Verification items for the finished model (mm, model axes). Face numbers are marked on the shaded views. A direction names the side the tool comes from. Give positions to 0.01 mm unless a question says otherwise; leave off trailing zeros. Loops run counter-clockwise (first coordinate to the right, second up) from the corner with the lowest first, then second, coordinate; pieces in that order, holes last. Notation, with made-up numbers: (15.25, 34) - (48.25, 34) arc R27 ccw to (48.25, 51) - close; hole circle Ø3 at (-16, -17). An arc over 180 degrees is marked (long way). One line per item, written item: value. Start each with the question number.
1. Mould release check, pull along Y, two halves, no side actions. Record for the marked faces 4, 5 and 6: pulls with the +Y half, pulls with the -Y half, needs draft (parallel to the pull), parting line crosses it, or undercut.
2. Sectioned sample at C-C (y = 28.5). Record the cut outline in (x, z), plus the area to 3 significant figures.
3. Sectioned sample at D-D (y = 18). Record the cut outline in (x, z).
4. Scan lines: L1, parallel to Z at x = 60, y = 20.5; L2, parallel to X at y = 4, z = 28; L3, parallel to Z at x = 39, y = 7.5. Record each from-to range of solid material in increasing order. Write a range as [from, to].
5. Access from +Z, -Z, +X, -X, +Y, -Y to the whole of each face (thin tool, end or side, straight path). Record for the marked faces 1, 2 and 3.
6. Gauge pin test, flat ends, axial feed: pin 1 (1 mm diameter, centred on x = 44.5, y = 35, fed in from +Z); pin 2 (9.5 mm diameter, centred on x = 54.5, y = 40.5, fed in from -Z); pin 3 (11 mm diameter, centred on x = 71.5, y = 18.5, fed in from -Z); pin 4 (6 mm diameter, centred on x = 12, y = 25, fed in from -Z). Record the tip position at first contact, or that the pin passes through.
7. Sectioned sample at A-A (x = 39). Record the cut outline in (y, z).
8. Sectioned sample at B-B (z = 28.5). Record the cut outline in (x, y).
from build123d import *

# Parameters (mm, degrees)
SKETCH1_W           = 68
SKETCH1_H           = 36.5
BOSS_EXTRUDE1_DEPTH = 6
SKETCH2_R           = 3.5
CUT_EXTRUDE1_DEPTH  = 78.409624725
SKETCH3_W           = 68
SKETCH3_H           = 4
BOSS_EXTRUDE2_DEPTH = 1
SKETCH4_R           = 5
SKETCH4_R_2         = 4
BOSS_EXTRUDE3_DEPTH = 4
FILLET1_R           = 2
SKETCH5_R           = 9.5
SKETCH5_R_2         = 4
SKETCH5_R_3         = 5
BOSS_EXTRUDE4_DEPTH = 1
FILLET2_R           = 2
CHAMFER1_SIZE       = 10
CHAMFER2_SIZE       = 16
FILLET3_R           = 2
SKETCH7_R           = 5
BOSS_EXTRUDE6_DEPTH = 18
SKETCH8_W           = 25
SKETCH8_H           = 25
CUT_EXTRUDE2_DEPTH  = 12
FILLET8_R           = 2
BOSS_EXTRUDE8_REACH = 99.236


with BuildPart() as part:
    # Sketch1 → Boss-Extrude1 (new body)
    with BuildSketch(Plane(origin=(0, 0, 0), x_dir=(1, 0, 0), z_dir=(0, 1, 0))):
        with Locations((34, 18.25)):
            Rectangle(SKETCH1_W, SKETCH1_H)
    boss_extrude1 = extrude(amount=BOSS_EXTRUDE1_DEPTH)

    # Sketch2 → Cut-Extrude1 (cut, through all)
    with BuildSketch(Plane(origin=(0, 6, 0), x_dir=(1, 0, 0), z_dir=(0, 1, 0))):
        with Locations(Location((12, 28.5, 0), (0, 0, 270))):
            Circle(SKETCH2_R)
        with Locations(Location((39, 28.5, 0), (0, 0, 270))):
            Circle(SKETCH2_R)
    cut_extrude1 = extrude(amount=-CUT_EXTRUDE1_DEPTH, mode=Mode.SUBTRACT)

    # Sketch3 → Boss-Extrude2 (add)
    with BuildSketch(Plane(origin=(0, 6, 0), x_dir=(1, 0, 0), z_dir=(0, 1, 0))):
        with Locations((34, 8)):
            Rectangle(SKETCH3_W, SKETCH3_H)
    boss_extrude2 = extrude(amount=BOSS_EXTRUDE2_DEPTH)

    # Sketch4 → Boss-Extrude3 (add)
    with BuildSketch(Plane.XY.offset(-6)):
        with BuildLine():
            Line((68, 6), (72.84831471, 18))
            Line((72.84831471, 18), (61.107812514, 47.058762637))
            ThreePointArc((61.107812514, 47.058762637), (47.739148723, 51.833822365), (44.553599203, 38))
            Line((44.553599203, 38), (0, 38))
            Line((0, 38), (0, 6))
            Line((0, 6), (68, 6))
        make_face()
        with Locations((12, 25)):
            Circle(SKETCH4_R, mode=Mode.SUBTRACT)
        with Locations((52.299565896, 43.5)):
            Circle(SKETCH4_R_2, mode=Mode.SUBTRACT)
    boss_extrude3 = extrude(amount=-BOSS_EXTRUDE3_DEPTH)

    # Mirror1: Boss-Extrude1, Cut-Extrude1, Boss-Extrude2, Boss-Extrude3 across plane
    add(boss_extrude1.mirror(Plane.XY))
    add(cut_extrude1.mirror(Plane.XY), mode=Mode.SUBTRACT)
    add(boss_extrude2.mirror(Plane.XY))
    add(boss_extrude3.mirror(Plane.XY))

    # Fillet1
    fillet1_edges = [part.edges().sort_by_distance(p)[0] for p in [
        (34, 6, -6),
        (34, 6, -10),
        (34, 6, 6),
        (34, 6, 10),
    ]]
    fillet(fillet1_edges, radius=FILLET1_R)

    # Sketch5 → Boss-Extrude4 (add)
    # profile 1 of 2: a face of its own
    with BuildSketch(Plane.XY.offset(10)):
        with Locations(Location((52.299565896, 43.5, 0), (0, 0, 215.376540152))):
            Circle(SKETCH5_R)
        with Locations((52.299565896, 43.5)):
            Circle(SKETCH5_R_2, mode=Mode.SUBTRACT)
    # profile 2 of 2: a face of its own
    with BuildSketch(Plane.XY.offset(10)):
        with Locations((12, 25)):
            Circle(SKETCH5_R)
        with Locations((12, 25)):
            Circle(SKETCH5_R_3, mode=Mode.SUBTRACT)
    boss_extrude4 = extrude(amount=BOSS_EXTRUDE4_DEPTH)

    # Fillet2
    # the kernel refuses this fillet: 2 mm, written as the material it adds along each edge
    with BuildSketch(Plane(origin=(44.553599203, 38, -6), x_dir=(-0.4469432732557111, 0.8945623010676621, 0), z_dir=(0, 0, -1))) as fillet2_piece_1:
        with BuildLine():
            CenterArc((3.223135148, -1.976302693), FILLET2_R, 98.828804139, 107.718931873)
            Line((1.434010546, -2.870189239), (0, 0))
            ThreePointArc((0, 0), (1.458084948, -0.112562209), (2.916169896, 0))
        make_face()
    extrude(amount=4)
    with BuildSketch(Plane(origin=(44.553599203, 38, 6), x_dir=(-0.4469432732557111, 0.8945623010676621, 0), z_dir=(0, 0, 1))) as fillet2_piece_2:
        with BuildLine():
            CenterArc((3.223135148, 1.976302693), FILLET2_R, 153.452263987, 107.718931873)
            Line((1.434010546, 2.870189239), (0, 0))
            ThreePointArc((0, 0), (1.458084948, 0.112562209), (2.916169896, 0))
        make_face()
    extrude(amount=4)
    # the kernel refuses this fillet: 2 mm, written as the material it takes off along each edge
    with BuildSketch(Plane(origin=(0, 38, -1), x_dir=(0, -1, 0), z_dir=(0, 0, -1))) as fillet2_2_piece_1:
        with BuildLine():
            CenterArc((FILLET2_R, -FILLET2_R), FILLET2_R, 90, 90)
            Line((0, -FILLET2_R), (0, 0))
            Line((0, 0), (FILLET2_R, 0))
        make_face()
    extrude(amount=14, mode=Mode.SUBTRACT)
    with BuildSketch(Plane(origin=(0, 38, 1), x_dir=(0, -1, 0), z_dir=(0, 0, 1))) as fillet2_2_piece_2:
        with BuildLine():
            CenterArc((FILLET2_R, FILLET2_R), FILLET2_R, 180, 90)
            Line((0, FILLET2_R), (0, 0))
            Line((0, 0), (FILLET2_R, 0))
        make_face()
    extrude(amount=14, mode=Mode.SUBTRACT)

    # Chamfer1
    chamfer1_edges = [part.edges().sort_by_distance(p)[0] for p in [
        (0, 3, 36.5),
        (0, 3, -36.5),
    ]]
    chamfer(chamfer1_edges, length=CHAMFER1_SIZE)

    # Chamfer2
    chamfer2_edges = [part.edges().sort_by_distance(p)[0] for p in [
        (68, 3, 36.5),
        (68, 3, -36.5),
    ]]
    chamfer(chamfer2_edges, length=CHAMFER2_SIZE)

    # Fillet3
    fillet3_edges = [part.edges().sort_by_distance(p)[0] for p in [
        (10, 3, 36.5),
        (0, 3, -26.5),
        (0, 3, 26.5),
        (10, 3, -36.5),
        (68, 3, -20.5),
        (68, 3, 20.5),
        (52, 3, 36.5),
        (52, 3, -36.5),
    ]]
    fillet(fillet3_edges, radius=FILLET3_R)

    # Mirror2: Boss-Extrude4 across plane
    add(boss_extrude4.mirror(Plane.XY))

    # Sketch7 → Boss-Extrude6 (add, symmetric)
    with BuildSketch(Plane.XY):
        with Locations((72.84831471, 18)):
            Circle(SKETCH7_R)
    extrude(amount=BOSS_EXTRUDE6_DEPTH, both=True)

    # Sketch8 → Cut-Extrude2 (cut)
    with BuildSketch(Plane(origin=(0, 0, 6), x_dir=(-1, 0, 0), z_dir=(0, 0, -1))):
        with Locations((-70.130356493, 22.5)):
            Rectangle(SKETCH8_W, SKETCH8_H)
    extrude(amount=CUT_EXTRUDE2_DEPTH, mode=Mode.SUBTRACT)

    # Fillet8
    fillet8_edges = [part.edges().sort_by_distance(p)[0] for p in [
        (70.975281743, 22.635919273, 8),
        (70.975281743, 13.364080727, -8),
        (70.975281743, 22.635919273, -8),
        (70.975281743, 13.364080727, 8),
    ]]
    fillet(fillet8_edges, radius=FILLET8_R)

    # Boss-Extrude8: up to this plane
    boss_extrude8_end = Plane(origin=(0, 6, 0), z_dir=(0, 1, 0))
    # Sketch11 → Boss-Extrude8 (add, up to the surface)
    with BuildSketch(Plane(origin=(0, 20.304963619, 11.723076211), x_dir=(-1, 0, 0), z_dir=(0, 0.866025403784438, 0.500000000000001)), mode=Mode.PRIVATE) as boss_extrude8_sk1:
        with BuildLine():
            Line((-6.5, 8.609927238), (-56.5, 8.609927238))
            ThreePointArc((-56.5, 8.609927238), (-59.5, 11.609927238), (-56.5, 14.609927238))
            Line((-56.5, 14.609927238), (-6.5, 14.609927238))
            ThreePointArc((-6.5, 14.609927238), (-3.5, 11.609927238), (-6.5, 8.609927238))
        make_face()
    boss_extrude8_tool1 = split(extrude(boss_extrude8_sk1.sketch, amount=-BOSS_EXTRUDE8_REACH, mode=Mode.PRIVATE), bisect_by=boss_extrude8_end, keep=Keep.BOTH, mode=Mode.PRIVATE)
    add(boss_extrude8_tool1.solids().sort_by_distance((31.5, 14.5, 21.777568))[0])


solid = part.part
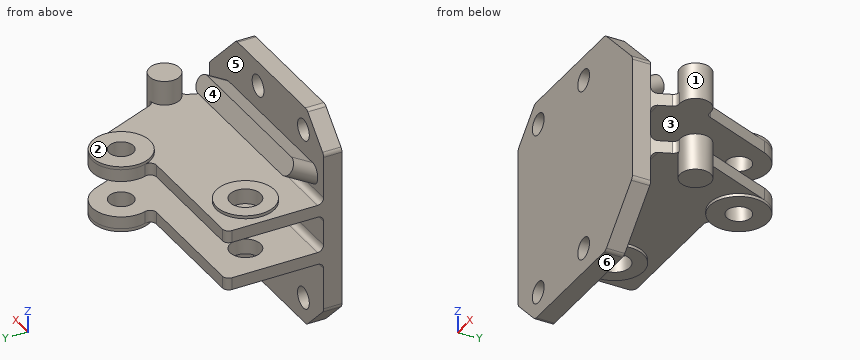
Results are:
1. face 4: pulls with the +Y half
1. face 5: undercut
1. face 6: needs draft
2. outline: (0, -10) - (3.17, -10) - (3.17, -11) - (8.43, -11) - (8.43, -6) - (0, -6) - close; (0, 6) - (8.43, 6) - (8.43, 11) - (3.17, 11) - (3.17, 10) - (0, 10) - close; (15.57, -11) - (20.83, -11) - (20.83, -10) - (68.61, -10) - (68.61, -6) - (15.57, -6) - close; (15.57, 6) - (68.61, 6) - (68.61, 10) - (20.83, 10) - (20.83, 11) - (15.57, 11) - close
2. area: 513 mm^2
3. outline: (0, -10) - (5.58, -10) - (5.58, -11) - (18.42, -11) - (18.42, -10) - (67.85, -10) - (67.85, -18) - (77.85, -18) - (77.85, -6) - (0, -6) - close; (0, 6) - (77.85, 6) - (77.85, 18) - (67.85, 18) - (67.85, 10) - (18.42, 10) - (18.42, 11) - (5.58, 11) - (5.58, 10) - (0, 10) - close
4. L1: z = [-10, -6], [6, 10]
4. L2: x = [1.5, 8.54], [15.46, 35.54], [42.46, 60.5]
4. L3: z = [-10.06, -5.94], [5.94, 10.06], [14.27, 21.2]
5. face 1: +Z
5. face 2: +Z, +X, -X, +Y
5. face 3: +X, -X, +Y
6. pin 1: stops at z = 10
6. pin 2: stops at z = -11
6. pin 3: stops at z = -18
6. pin 4: passes through
7. outline: (0, -36.5) - (6, -36.5) - (6, -32) - (0, -32) - close; (0, -25) - (6, -25) - (6, -12) arc R2 cw to (8, -10) - (38, -10) - (38, -6) - (8, -6) arc R2 cw to (6, -4) - (6, 4) arc R2 cw to (8, 6) - (38, 6) - (38, 10) - (8, 10) arc R2 cw to (6, 12) - (6, 13.41) - (16, 19.18) - (13, 24.38) - (6, 20.33) - (6, 25) - (0, 25) - close; (0, 32) - (6, 32) - (6, 36.5) - (0, 36.5) - close
8. outline: (2, 0) - (8.5, 0) - (8.5, 6) - (2, 6) - close; (15.5, 0) - (35.5, 0) - (35.5, 6) - (15.5, 6) - close; (42.5, 0) - (60, 0) - (60, 6) - (42.5, 6) - close
